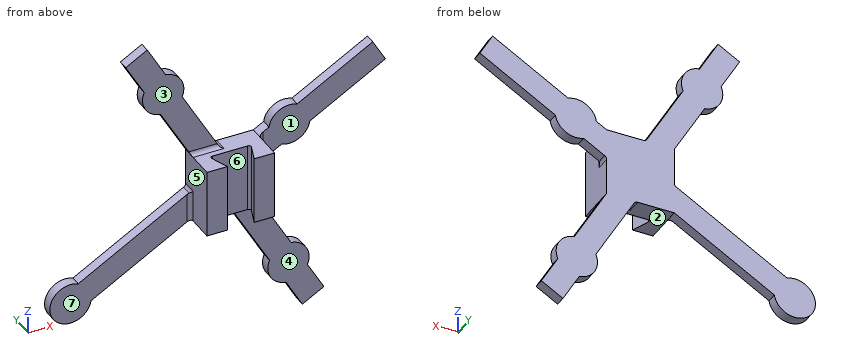
Autodesk Inventor part; units mm, degrees
ref_plane "YZ Plane" through (0, 0, 0) normal (1, 0, 0) x (0, 1, 0)
ref_plane "XZ Plane" through (0, 0, 0) normal (0, 1, 0) x (-1, 0, 0)
ref_plane "XY Plane" through (0, 0, 0) normal (0, 0, 1) x (1, 0, 0)
sketch "Sketch1" plane through (0, 0, 0) normal (0, 0, 1) x (1, 0, 0)
  line L0 (0, 5) -> (4.285926, 5)
  line L1 (4.755772, 4.32899) -> (3.180149, 0)
  line L2 (3.180149, 0) -> (0, 0)
  line L3 (0, 5) -> (-4.285926, 5)
  line L4 (-4.755772, 4.32899) -> (-3.180149, 0)
  line L5 (-3.180149, 0) -> (0, 0)
  arc A0 (-4.285926, 5) -> (-4.755772, 4.32899) centre (-4.285926, 4.5) ccw
  arc A1 (4.755772, 4.32899) -> (4.285926, 5) centre (4.285926, 4.5) ccw
  line L6 (4.285926, 5.05) -> (0, 5.05)
  line L7 (0, 5.05) -> (-4.285926, 5.05)
  arc A2 (-4.285926, 5.05) -> (-4.802757, 4.311889) centre (-4.285926, 4.5) ccw
  line L8 (-4.802757, 4.311889) -> (-3.215159, -0.05)
  line L9 (-3.215159, -0.05) -> (0, -0.05)
  line L10 (0, -0.05) -> (3.215159, -0.05)
  line L11 (3.215159, -0.05) -> (4.802757, 4.311889)
  arc A3 (4.802757, 4.311889) -> (4.285926, 5.05) centre (4.285926, 4.5) ccw
  line L12 (-3.180149, 0) -> (-8.180149, 0)
  line L13 (-8.180149, 0) -> (-8.180149, 7.5)
  line L14 (3.180149, 0) -> (8.180149, 0)
  line L15 (8.180149, 0) -> (8.180149, 7.5)
  line L16 (8.180149, 7.5) -> (-8.180149, 7.5)
  point P0 (5, 5)
  point P1 (-5, 5)
  point P2 (3.233358, 0)
  point P3 (-3.233358, 0)
  dimension "d0" = 5
  dimension "d1" = 5
  dimension "d2" = 70
  dimension "d3" = 5
  dimension "d4" = 70
  dimension "d5" = 0.5
  dimension "d6" = 0.05
  dimension "d7" = 5
  dimension "d8" = 7.5
  dimension "d9" = 5
extrude "Extrusion1" add sketch "Sketch1" along normal blind 16.5 contours L11 A3 L6 L7 A2 L8 L12 L13 L16 L15 L14
sketch "Sketch2" plane through (-8.180149, 7.5, 0) normal (0, 1, 0) x (1, 0, 0)
  line L0 (-10.580957, -47.057485) -> (32.148268, 27.576377)
  line L1 (32.148268, 27.576377) -> (26.941254, 30.557485)
  line L2 (26.941254, 30.557485) -> (-15.78797, -44.076377)
  line L3 (-15.78797, -44.076377) -> (-10.580957, -47.057485)
  line L4 (-10.580957, -47.057485) -> (26.941254, 30.557485) construction
  line L5 (32.148268, 27.576377) -> (-15.78797, -44.076377) construction
  circle A0 centre (-6.725395, -34.285068) radius 5
  circle A1 centre (23.582544, 18.652904) radius 5
  line L6 (-13.184463, -45.566931) -> (29.544761, 29.066931) construction
  line L7 (16.360298, -16.5) -> (0, -16.5) construction
  line L8 (0, 0) -> (16.360298, -16.5) construction
  line L9 (16.360298, 0) -> (0, 0) construction
  line L10 (16.360298, -16.5) -> (16.360298, 0) construction
  line L11 (16.360298, 0) -> (0.368439, -15.856459) construction
  line L12 (-30.674699, 10.428379) -> (-27.598866, 15.800845)
  line L13 (-27.598866, 15.800845) -> (47.034997, -26.928379)
  line L14 (47.034997, -26.928379) -> (43.959163, -32.300845)
  line L15 (43.959163, -32.300845) -> (-30.674699, 10.428379)
  line L16 (-30.674699, 10.428379) -> (47.034997, -26.928379) construction
  line L17 (-27.598866, 15.800845) -> (43.959163, -32.300845) construction
  circle A2 centre (-29.136782, 13.114612) radius 5
  circle A3 centre (23.80119, -17.193326) radius 5
  line L18 (-29.136782, 13.114612) -> (45.49708, -29.614612)
  point P0 (8.180149, 0)
  point P1 (8.180149, -8.25)
  point P2 (8.180149, -8.25)
  point P3 (-24.191137, 13.849859)
  point P4 (-27.26697, 8.477393)
  point P5 (4.038725, -9.445679)
  point P6 (-7.341496, -29.323171)
  point P7 (-11.316307, -36.265856)
  point P8 (-6.109293, -39.246965)
  point P9 (-2.134482, -32.30428)
  point P10 (9.245739, -12.426788)
  point P11 (18.855544, -17.928573)
  point P12 (25.671002, -21.830545)
  point P13 (28.746835, -16.458079)
  point P14 (21.931377, -12.556107)
  point P15 (12.321572, -7.054321)
  point P16 (24.198645, 13.691007)
  point P17 (28.173456, 20.633692)
  point P18 (22.966443, 23.614801)
  point P19 (18.991631, 16.672116)
  point P20 (7.114559, -4.073212)
  dimension "d12" = 86
  dimension "d13" = 6
  dimension "d14" = 10
  dimension "d15" = 10
  dimension "d16" = 61
  dimension "d17" = 12
  dimension "d19" = 86
  dimension "d20" = 10
  dimension "d21" = 10
  dimension "d22" = 61
  dimension "d26" = 90
extrude "Extrusion2" add sketch "Sketch2" along normal blind 2.5
sketch "Sketch3" plane through (-8.180149, 7.5, 0) normal (0, 1, 0) x (1, 0, 0)
  line L0 (0, -7.133436) -> (0, -16.5)
  line L1 (9.446546, 0) -> (0, 0)
  line L2 (16.360298, 0) -> (16.360298, -9.366564)
  line L3 (16.360298, -16.5) -> (6.913752, -16.5)
  line L4 (0, 0) -> (4.946791, 0)
  line L5 (0, 0) -> (16.360298, 0)
  line L6 (16.360298, 0) -> (16.360298, -16.5)
  line L7 (16.360298, -16.5) -> (0, -16.5)
  line L8 (0, -16.5) -> (0, 0)
  point P0 (8.180149, 0)
  point P1 (0, -16.418433)
  point P2 (16.360298, -0.081567)
  point P3 (0, -16.418433)
  point P4 (16.360298, -0.081567)
extrude "Extrusion3" add sketch "Sketch3" along normal blind 2.5
fillet "Fillet1" radius 1 8 edges at (4.7233, 7.5, 0) (1.2664, 8.75, 0) (-8.1801, 7.5, 3.5667) (-8.1801, 8.75, 7.1334) (-4.7233, 7.5, 16.5) (-1.2664, 8.75, 16.5) (8.1801, 7.5, 12.9333) (8.1801, 8.75, 9.3666)
properties part number "female1"
The listing builds one solid part. Answer for the finished solid, in the listing's coordinates (mm). Face numbers are marked on the shaded views. A direction names the side the tool comes from. Coordinates: 2 decimals unless noted, no trailing zeros. Write each loop counter-clockwise with the first axis right and the second up, starting at its lowest first coordinate (ties: lowest second). Pieces come first, ordered by that corner, then holes. Notation, with made-up numbers: (74, 13) - (98, 13) arc R6 ccw to (98, 23) - close; hole circle Ø9 at (-25.75, -35). An arc over 180 degrees is marked (long way). Return JSON: item names as keys, results as strings. Group by question number.
Q1. Find the intervals of material crossed by line 1 along Y through (x, z) = (17.5, 19.5); line 2 along X through (y, z) = (9.25, 23); line 3 along Z through (x, y) = (6.5, 6.25), in increasing order. Write a range as [from, to].
Q2. For a pull along X with two mould halves and no side action, classify the marked faces 5, 6 and 7 as +X half, -X half, draft (parallel to the pull), parting line (faces both ways), or undercut.
Q3. Which of the six approach directions +Z, -Z, +X, -X, +Y, -Y give full straight-line access (tool end or side, diameter ignored) to the marked faces 1, 2, 3 and 4?
Q4. The part is cut by section D-D on z = 3. Write down the section's boundary in (x, y).
Q5. Flat-ended cylindrical pins translate along their axes: pin 1 Ø6 at (x, y) = (10.5, 3) entering from -Z; pin 2 Ø3 at (x, z) = (29, 24) entering from -Y; pin 3 Ø9.5 at (x, z) = (-2, 4.5) entering from -Y; pin 4 Ø6 at (x, y) = (-7.5, 4.5) entering from -Z. Find the tip coordinate at first contact, or state that the pin passes through.
Q6. The part is cut by section A-A on y = 1. Write down the section's boundary in (x, z).
Q7. The part is cut by section B-B on x = -22. Write down the section's boundary in (y, z).
Evaluation:
{
 "1": {"line 1": "y = [7.5, 10]", "line 2": "x = [-11.9, -4.99], [19.53, 31.99]", "line 3": "z = [0, 16.5]"},
 "2": {"face 5": "-X half", "face 6": "undercut", "face 7": "draft"},
 "3": {"face 1": "+Z, -Z, +X, -Y", "face 2": "-Z, -Y", "face 3": "+Z, +X, -X, -Y", "face 4": "-Z, +X, -X, -Y"},
 "4": {"outline": "(-15.4, 7.5) - (-9.18, 7.5) arc R1 cw to (-8.18, 6.5) - (-8.18, 0) - (-3.23, 0) - (-4.8, 4.31) arc R0.55 cw to (-4.29, 5.05) - (4.29, 5.05) arc R0.55 cw to (4.8, 4.31) - (3.23, 0) - (8.18, 0) - (8.18, 10) - (-15.4, 10) - close"},
 "5": {"pin 1": "stops at z = 0", "pin 2": "stops at y = 7.5", "pin 3": "stops at y = 0", "pin 4": "stops at z = -0.23"},
 "6": {"outline": "(-8.18, 0) - (-3.6, 0) - (-3.6, 16.5) - (-8.18, 16.5) - close; (3.6, 0) - (8.18, 0) - (8.18, 16.5) - (3.6, 16.5) - close"},
 "7": {"outline": "(7.5, -7.91) - (10, -7.91) - (10, -0.78) - (7.5, -0.78) - close; (7.5, 40.64) - (10, 40.64) - (10, 45.2) - (7.5, 45.2) - close"}
}
